Autodesk Inventor part; units mm, degrees
ref_plane "YZ Plane" through (0, 0, 0) normal (1, 0, 0) x (0, 1, 0)
ref_plane "XZ Plane" through (0, 0, 0) normal (0, 1, 0) x (-1, 0, 0)
ref_plane "XY Plane" through (0, 0, 0) normal (0, 0, 1) x (1, 0, 0)
sketch "Skizze1" plane through (0, 0, 0) normal (0, 0, 1) x (1, 0, 0)
  line L0 (-14, 6.25) -> (-5, 6.25)
  line L1 (-4, 5.25) -> (-4, -5.25)
  line L2 (-5, -6.25) -> (-14, -6.25)
  line L3 (-15, -5.25) -> (-15, 5.25)
  line L4 (-15, 6.25) -> (-4, -6.25) construction
  line L5 (-4, 6.25) -> (-15, -6.25) construction
  line L6 (6.5, 6.25) -> (14, 6.25)
  line L7 (15, 5.25) -> (15, -5.25)
  line L8 (14, -6.25) -> (6.5, -6.25)
  line L9 (5.5, -5.25) -> (5.5, 5.25)
  line L10 (5.5, 6.25) -> (15, -6.25) construction
  line L11 (15, 6.25) -> (5.5, -6.25) construction
  arc A0 (-15, -5.25) -> (-14, -6.25) centre (-14, -5.25) ccw
  arc A1 (-14, 6.25) -> (-15, 5.25) centre (-14, 5.25) ccw
  arc A2 (-4, 5.25) -> (-5, 6.25) centre (-5, 5.25) ccw
  arc A3 (-5, -6.25) -> (-4, -5.25) centre (-5, -5.25) ccw
  arc A4 (6.5, 6.25) -> (5.5, 5.25) centre (6.5, 5.25) ccw
  arc A5 (15, 5.25) -> (14, 6.25) centre (14, 5.25) ccw
  arc A6 (14, -6.25) -> (15, -5.25) centre (14, -5.25) ccw
  arc A7 (5.5, -5.25) -> (6.5, -6.25) centre (6.5, -5.25) ccw
  line L12 (-4, 4.5) -> (5.5, 4.5)
  line L13 (5.5, 4.5) -> (5.5, -4.5)
  line L14 (5.5, -4.5) -> (-4, -4.5)
  line L15 (-4, -4.5) -> (-4, 4.5)
  circle A8 centre (0, 0) radius 20
  line L16 (-15.25, -6.75) -> (15.25, -6.75)
  line L17 (15.25, -6.75) -> (15.25, 6.75)
  line L18 (15.25, 6.75) -> (-15.25, 6.75)
  line L19 (-15.25, 6.75) -> (-15.25, -6.75)
  line L20 (-15.25, -6.75) -> (15.25, 6.75) construction
  line L21 (15.25, -6.75) -> (-15.25, 6.75) construction
  line L22 (0, 6.75) -> (0, -6.75) construction
  line L23 (-28, 0) -> (28, 0)
  circle A9 centre (0, 0) radius 15 construction
  line L24 (10.6066, 10.6066) -> (-10.6066, -10.6066) construction
  line L25 (-10.6066, 10.6066) -> (10.6066, -10.6066) construction
  line L26 (6, 20) -> (-4.5, 20)
  line L27 (-4.5, 20) -> (-4.5, 4.5)
  line L28 (-4.5, 4.5) -> (6, 4.5)
  line L29 (6, 4.5) -> (6, 20)
  line L30 (20, 4) -> (15.25, 4)
  line L31 (15.25, 4) -> (15.25, -4)
  line L32 (15.25, -4) -> (20, -4)
  line L33 (20, -4) -> (20, 4)
  line L34 (-15.25, 4) -> (-20, 4)
  line L35 (-20, 4) -> (-20, -4)
  line L36 (-20, -4) -> (-15.25, -4)
  line L37 (-15.25, -4) -> (-15.25, 4)
  point P0 (-9.5, 0)
  point P1 (10.25, 0)
  point P2 (-9.5, 0)
  point P3 (10.25, 0)
  point P4 (-9.5, 0)
  point P5 (-4, 0)
  point P6 (5.5, 0)
  point P7 (10.25, 0)
  point P8 (0.75, 4.5)
  point P9 (0, 0)
  point P10 (0.75, 20)
  dimension "d5" = 12.5
  dimension "d6" = 11
  dimension "d7" = 9.5
  dimension "d9" = 1
  dimension "d10" = 1
  dimension "d12" = 9
  dimension "d14" = 40
  dimension "d15" = 13.5
  dimension "d16" = 30.5
  dimension "d17" = 30
  dimension "d18" = 9.5
  dimension "d47" = 30
  dimension "d48" = 90
  dimension "d49" = 45
  dimension "d50" = 10.5
  dimension "d55" = 8
extrude "Extrusion1" add sketch "Skizze1" along normal blind 194.899 contours A1 L3 L23 L19 L18 L27 A2 L0 | L27 L18 L29 A4 L9 L12 L1 A2 | L3 A0 L2 A3 L1 L14 L9 A7 L8 A6 L7 L23 L17 L16 L19 | L27 A8 L29 L18 | L18 L19 L34 A8 L27 | L23 A8 L34 L19 | L19 L36 A8 L23 | L23 L9 L14 L1 | L1 L12 L9 L23 | L29 A8 L30 L17 L18 | L18 L17 L23 L7 A5 L6 A4 L29 | L19 L16 L17 L32 A8 L36 | L30 A8 L23 L17 | L32 L17 L23 A8
extrude "Extrusion4" cut sketch "Skizze1" along normal blind 10 contours A1 L3 L23 L19 L18 L27 A2 L0 | L27 L18 L29 A4 L9 L12 L1 A2 | A2 L1 L28 L27 | L3 A0 L2 A3 L1 L14 L9 A7 L8 A6 L7 L23 L17 L16 L19 | L27 A8 L29 L18 | L23 L9 L14 L1 | L1 L12 L9 L23 | L18 L17 L23 L7 A5 L6 A4 L29 | L27 L26 A8 | L9 A4 L29 L28 | A8 L26 L29
extrude "Extrusion6" cut sketch "Skizze1" along normal blind 17 contours L23 L9 L14 L1 | L1 L12 L9 L23
extrude "Extrusion5" cut sketch "Skizze1" along normal blind 6 contours L23 A8 L34 L19 | L19 L36 A8 L23 | L35 L34 A8 | A8 L36 L35 | L30 A8 L23 L17 | L30 L33 A8 | L32 L17 L23 A8 | A8 L33 L32
sketch "Skizze2" plane through (0, 0, 194.899) normal (0, 0, 1) x (1, 0, 0)
  arc A0 (-15, -5.25) -> (-14, -6.25) centre (-14, -5.25) ccw
  line L0 (-15, -5.25) -> (-15, 5.25)
  arc A1 (-14, 6.25) -> (-15, 5.25) centre (-14, 5.25) ccw
  line L1 (-14, 6.25) -> (-5, 6.25)
  arc A2 (-4, 5.25) -> (-5, 6.25) centre (-5, 5.25) ccw
  line L2 (-4, 5.25) -> (-4, -5.25)
  arc A3 (-5, -6.25) -> (-4, -5.25) centre (-5, -5.25) ccw
  line L3 (-5, -6.25) -> (-14, -6.25)
  arc A4 (6.5, 6.25) -> (5.5, 5.25) centre (6.5, 5.25) ccw
  line L4 (6.5, 6.25) -> (14, 6.25)
  arc A5 (15, 5.25) -> (14, 6.25) centre (14, 5.25) ccw
  line L5 (15, 5.25) -> (15, -5.25)
  arc A6 (14, -6.25) -> (15, -5.25) centre (14, -5.25) ccw
  line L6 (14, -6.25) -> (6.5, -6.25)
  arc A7 (5.5, -5.25) -> (6.5, -6.25) centre (6.5, -5.25) ccw
  line L7 (5.5, -5.25) -> (5.5, 5.25)
  circle A8 centre (0, 0) radius 20
  line L8 (-50, -50) -> (50, -50)
  line L9 (50, -50) -> (50, 50)
  line L10 (50, 50) -> (-50, 50)
  line L11 (-50, 50) -> (-50, -50)
  line L12 (-50, -50) -> (50, 50) construction
  line L13 (50, -50) -> (-50, 50) construction
  line L14 (-48.8, 48.8) -> (48.8, 48.8)
  line L15 (48.8, 48.8) -> (48.8, -48.8)
  line L16 (48.8, -48.8) -> (-48.8, -48.8)
  line L17 (-48.8, -48.8) -> (-48.8, 48.8)
  dimension "d19" = 100
  dimension "d20" = 100
  dimension "d21" = 1.2
extrude "Extrusion2" add sketch "Skizze2" along normal blind 2 contours A8 | L11 L10 L9 L8 | L14 L15 L16 L17
extrude "Extrusion3" add sketch "Skizze2" against normal blind 2 contours L14 L15 L16 L17
hole "Bohrung1" at (10.6066, 10.6066, 0) at (-10.6066, 10.6066, 0) at (-10.6066, -10.6066, 0) at (10.6066, -10.6066, 0) direction (0, 0, 1) diameter 2.2 depth 5
sketch "Skizze3" plane through (0, 0, 0) normal (0, 1, 0) x (-1, 0, 0)
  line L0 (20, 12) -> (20.5, 12)
  line L1 (20.5, 12) -> (20.5, 0)
  line L2 (20.5, 0) -> (20, 0)
  line L3 (20, 0) -> (20, 12)
  line L4 (20.6, 0) -> (19.9, 0)
  line L5 (0, -2.4) -> (0, 14.4)
  dimension "d26" = 12
  dimension "d27" = 0.5
  dimension "d37" = 40
equation "\"d20\" = d19"
properties part number "DayLightGlow_Rod"
Here's how the part is built. I have some questions about the finished solid (model axes, mm). A direction names the side the tool comes from. Coordinates: 2 decimals unless noted, no trailing zeros. Order: outer loops, then holes, each group sorted by start corner. A loop starts at its lowest first (then second) coordinate and runs counter-clockwise, first axis right, second up.
1) Imagine slicing it at D-D on x = 0. List the corners of the cut face in (y, z) for me.
2) We'd pull the mould along Y, two halves only. Please class faces 5 (the face through (11, 12, 0)), 6 (the face through (17, 4, 3)), 7 (the face through (18, 0, 6)), 8 (the face through (10.752, -16.864, 95.099)): +Y half, -Y half, draft (parallel to the pull), parting line (faces both ways), or undercut.
3) Imagine slicing it at C-C on x = 25. List the corners of the cut face in (y, z) for me, and give its area (3 significant figures).
4) I need wall thicknesses on line 1 (X direction, y = -4, z = 85.5); line 2 (Z direction, x = -40, y = 17.5); line 3 (X direction, y = -5, z = 97.5). Which ranges of each line are inside material? Lowest first, please.
5) Imagine slicing it at B-B on z = 146.5. List the corners of the cut face in (x, y) for me, and give its area (3 significant figures).
6) Imagine slicing it at A-A on y = 0. List the corners of the cut face in (x, z) for me, and give its area (3 significant figures).
7) Which directions (+Z, -Z, +X, -X, +Y, -Y) give clear straight access to the entire face, cutting with the end or side of a thin tool? Please do faces 1 (the face through (-10, 12, 0)), 2 (the face through (-10, 6.25, 102)), 3 (the face through (-10, 6.75, 5)), 4 (the face through (-17, 4, 3)).
8) Will these pins go through, and if not, where does the flat tip stop? pin 1 (12 mm diameter, centred on x = 10.5, z = 71, fed in from +Y); pin 2 (5.5 mm diameter, centred on x = -1, z = 13.5, fed in from -Y); pin 3 (4 mm diameter, centred on x = 11.5, z = 93.5, fed in from +Y).
Response values:
1. outline: (-50, 194.9) - (-48.8, 194.9) - (-48.8, 192.9) - (-20, 192.9) - (-20, 0) - (-6.75, 0) - (-6.75, 10) - (-4.5, 10) - (-4.5, 17) - (4.5, 17) - (4.5, 10) - (20, 10) - (20, 192.9) - (48.8, 192.9) - (48.8, 194.9) - (50, 194.9) - (50, 196.9) - (-50, 196.9) - close
2. face 5: draft
2. face 6: undercut
2. face 7: undercut
2. face 8: parting line
3. outline: (-50, 194.9) - (-48.8, 194.9) - (-48.8, 192.9) - (48.8, 192.9) - (48.8, 194.9) - (50, 194.9) - (50, 196.9) - (-50, 196.9) - close
3. area: 395 mm2
4. line 1: x = -19.6 to -15, -4 to 5.5, 15 to 19.6
4. line 2: z = 192.9 to 196.9
4. line 3: x = -19.36 to -15, -4 to 5.5, 15 to 19.36
5. outline: circle Ø40 at (0, 0); hole (-15, -5.25) arc R1 ccw to (-14, -6.25) - (-5, -6.25) arc R1 ccw to (-4, -5.25) - (-4, 5.25) arc R1 ccw to (-5, 6.25) - (-14, 6.25) arc R1 ccw to (-15, 5.25) - close; hole (5.5, -5.25) arc R1 ccw to (6.5, -6.25) - (14, -6.25) arc R1 ccw to (15, -5.25) - (15, 5.25) arc R1 ccw to (14, 6.25) - (6.5, 6.25) arc R1 ccw to (5.5, 5.25) - close
5. area: 1,000 mm2
6. outline: (-50, 194.9) - (-48.8, 194.9) - (-48.8, 192.9) - (-20, 192.9) - (-20, 6) - (-15.25, 6) - (-15.25, 10) - (-15, 10) - (-15, 196.9) - (-50, 196.9) - close; (-4, 17) - (5.5, 17) - (5.5, 196.9) - (-4, 196.9) - close; (15, 10) - (15.25, 10) - (15.25, 6) - (20, 6) - (20, 192.9) - (48.8, 192.9) - (48.8, 194.9) - (50, 194.9) - (50, 196.9) - (15, 196.9) - close
6. area: 3,850 mm2
7. face 1: -Z, +X, -X, +Y, -Y
7. face 2: +Z, -Z
7. face 3: -Z
7. face 4: -Z, +X, -X
8. pin 1: stops at y = 19.49
8. pin 2: stops at y = -20
8. pin 3: stops at y = 17.6
